Input: part model. Units: mm. Frame: model coordinates. A direction names the side the tool comes from. Round coordinates to 2 decimals unless told otherwise and drop trailing zeros. Loops run counter-clockwise (first coordinate to the right, second up) from the corner with the lowest first, then second, coordinate; pieces in that order, holes last. Notation, with made-up numbers: (12, -0.5) - (27, -0.5) arc R18 ccw to (27, 5.5) - close; hole circle Ø2 at (62, 70.25). An arc over 180 degrees is marked (long way). One line per question, with ' | ' between items. Start each with the question number.
Item 1: Material intervals for line 1 along Y through (x, z) = (2, 56); line 2 along Y through (x, z) = (1.35, 32.5); line 3 along Z through (x, y) = (2, 15), sorted ascending.
Item 2: Section A-A, the plane y = 39. Return loops of the section in (x, z), plus the area to 3 significant figures.
Item 3: Section B-B, the plane z = 56. Return loops of the section in (x, y).
Item 4: First-contact query: pin 1 (23 mm diameter, centred on y = 39, z = 32.5, fed in from +X); pin 2 (19.5 mm diameter, centred on x = 43.5, z = 28, fed in from +Y); pin 3 (19.5 mm diameter, centred on y = 48, z = 24, fed in from +X). Flat tips, straight axial feed; report the tip coordinate or a pass-through.
Item 5: Section C-C, the plane z = 24.5. Return loops of the section in (x, y).
Item 6: Section D-D, the plane y = 15.5. Return loops of the section in (x, z).
Item 7: Draft query along Z for faces 1 (the face through (39, 1, 50.25)), 2 (the face through (11.38, 16.69, 0.99)), 3 (the face through (1, 65, 62)), 4 (the face through (35, 3, 32)). Return one class per face: pulls with the +Z half, pulls with the -Z half, needs draft (parallel to the pull), parting line crosses it, or undercut.
Item 8: Set-up query: faces 5 (the face through (9, 11, 63)), 6 (the face through (39, 1, 10.25)), 7 (the face through (65, 2, 3)). Return all of +Z, -Z, +X, -X, +Y, -Y with unobstructed straight access to the full face (end or side cutting, diameter ignored); none if empty.
```python
from build123d import *

# Parameters (mm, degrees)
EXTRUDE_1_DEPTH             = 65
HOLE_WIZARD_4_5_4_5_1_DEPTH = 3
SKETCH_4_R                  = 19
CUT_EXTRUDE_1_DEPTH         = 65
HOLE_WIZARD_5_0_5_1_D       = 5
CHAMFER_1_SIZE              = 6
RIB_18_REACH                = 118.073
SKETCH_9_WALL_W             = 266.052617732
SKETCH_9_WALL_H             = 2
RIB_19_REACH                = 118.073
SKETCH_8_WALL_W             = 266.052617732
SKETCH_8_WALL_H             = 2


# Read off the part's stored shape, not the designer's step: Ø4.5 (4.5) 直径槽口1
with BuildPart() as part:
    # 草图1 → 凸台-拉伸1 (new body)
    with BuildSketch(Plane.XY):
        Polygon((0, 0), (0, 68), (3, 68), (3, 3), (68, 3), (68, 0), align=None)
    extrude(amount=EXTRUDE_1_DEPTH)

    # Ø4.5 (4.5) 直径槽口1 outline → Ø4.5 (4.5) 直径槽口1 (cut)
    with BuildSketch(Plane(origin=(0, 0, 0), x_dir=(1, 0, 0), z_dir=(0, 1, 0))):
        with BuildLine():
            Line((18.25, -14.75), (58.75, -14.75))
            ThreePointArc((58.75, -14.75), (61, -12.5), (58.75, -10.25))
            Line((58.75, -10.25), (18.25, -10.25))
            ThreePointArc((18.25, -10.25), (16, -12.5), (18.25, -14.75))
        make_face()
        with BuildLine():
            Line((18.25, -54.75), (58.75, -54.75))
            ThreePointArc((58.75, -54.75), (61, -52.5), (58.75, -50.25))
            Line((58.75, -50.25), (18.25, -50.25))
            ThreePointArc((18.25, -50.25), (16, -52.5), (18.25, -54.75))
        make_face()
    extrude(amount=HOLE_WIZARD_4_5_4_5_1_DEPTH, mode=Mode.SUBTRACT)

    # 草图4 → 切除-拉伸1 (cut)
    with BuildSketch(Plane.ZY):
        with Locations((32.5, 39)):
            Circle(SKETCH_4_R)
    extrude(amount=-CUT_EXTRUDE_1_DEPTH, mode=Mode.SUBTRACT)

    # Ø5.0 (5) 直径孔1 (through all)
    with Locations(Plane.ZY):
        with Locations((9, 62.5), (56, 62.5), (9, 15.5), (56, 15.5)):
            Hole(HOLE_WIZARD_5_0_5_1_D / 2)

    # 倒角1
    chamfer_1_edges = [part.edges().sort_by_distance(p)[0] for p in [
        (1.5, 68, 65),
        (1.5, 68, 0),
        (68, 1.5, 65),
        (68, 1.5, 0),
    ]]
    chamfer(chamfer_1_edges, length=CHAMFER_1_SIZE)

    # 草图9 wall → 筋18 (add, up to next)
    with BuildSketch(Plane(origin=(11.5, 16.5, 0), x_dir=(0.532813269686, -0.84623284009, 0), z_dir=(0.84623284009, 0.532813269686, 0)), mode=Mode.PRIVATE) as rib_18_sk1:
        with Locations((0, -1)):
            Rectangle(SKETCH_9_WALL_W, SKETCH_9_WALL_H)
    rib_18_tool1 = extrude(rib_18_sk1.sketch, amount=-RIB_18_REACH, mode=Mode.PRIVATE) - part.part
    add(rib_18_tool1.solids().sort_by_distance((11.5, 16.5, 0))[0])

    # 草图8 wall → 筋19 (add, up to next)
    with BuildSketch(Plane(origin=(11.5, 16.5, 65), x_dir=(0.532813269686, -0.84623284009, 0), z_dir=(0.84623284009, 0.532813269686, 0)), mode=Mode.PRIVATE) as rib_19_sk1:
        with Locations((0, 1)):
            Rectangle(SKETCH_8_WALL_W, SKETCH_8_WALL_H)
    rib_19_tool1 = extrude(rib_19_sk1.sketch, amount=-RIB_19_REACH, mode=Mode.PRIVATE) - part.part
    add(rib_19_tool1.solids().sort_by_distance((11.5, 16.5, 65))[0])


solid = part.part
```
Return value:
1) line 1: 0 to 13, 18 to 60, 65 to 68 | line 2: 0 to 20, 58 to 68 | line 3: 0 to 6.55, 11.45 to 53.55, 58.45 to 65
2) outline: (0, 0) - (3, 0) - (3, 13.5) - (0, 13.5) - close; (0, 51.5) - (3, 51.5) - (3, 65) - (0, 65) - close | area: 81.0 mm2
3) outline: (0, 0) - (68, 0) - (68, 3) - (3, 3) - (3, 13) - (0, 13) - close; (0, 18) - (3, 18) - (3, 60) - (0, 60) - close; (0, 65) - (3, 65) - (3, 68) - (0, 68) - close
4) pin 1: through | pin 2: y = 3 | pin 3: x = 3
5) outline: (0, 0) - (68, 0) - (68, 3) - (3, 3) - (3, 21.77) - (0, 21.77) - close; (0, 56.23) - (3, 56.23) - (3, 68) - (0, 68) - close
6) outline: (0, 0) - (12.13, 0) - (12.13, 2) - (3, 2) - (3, 6.5) - (0, 6.5) - close; (0, 11.5) - (3, 11.5) - (3, 53.5) - (0, 53.5) - close; (0, 58.5) - (3, 58.5) - (3, 63) - (12.13, 63) - (12.13, 65) - (0, 65) - close
7) face 1: undercut | face 2: needs draft | face 3: pulls with the +Z half | face 4: undercut
8) face 5: +X, +Y | face 6: +Y, -Y | face 7: -Z, +X, +Y, -Y
